Autodesk Inventor part; units mm, degrees
ref_plane "Work Plane1" through (6, 0, 0) normal (1, 0, 0) x (0, 0, -1)
ref_plane "YZ Plane" through (0, 0, 0) normal (1, 0, 0) x (0, 1, 0)
ref_plane "XZ Plane" through (0, 0, 0) normal (0, 1, 0) x (-1, 0, 0)
sketch "Sketch2" plane through (0, 0, 0) normal (1, 0, 0) x (0, 1, 0)
  line L0 (0, 0) -> (15, 0)
  line L1 (15, 0) -> (15, -10)
  line L2 (15, -10) -> (0, -10)
  line L3 (0, -10) -> (0, 0)
  dimension "d4" = 15
  dimension "d5" = 10
extrude "Extrusion2" add sketch "Sketch2" along normal blind 12
sketch "Sketch3" plane through (0, 0, 0) normal (0, 0, 1) x (1, 0, 0)
  line L0 (0, 0) -> (1, 0)
  line L1 (0, 0) -> (12, 0)
  line L2 (1, 0) -> (1, 13.5)
  line L3 (1, 13.5) -> (11, 13.5)
  line L4 (11, 13.5) -> (11, 0)
  line L5 (11, 0) -> (1, 0)
  dimension "d8" = 1
  dimension "d9" = 13.5
  dimension "d10" = 10
extrude "Extrusion3" cut sketch "Sketch3" against normal blind 8
sketch "Sketch4" plane through (0, 0, -10) normal (0, 0, -1) x (-1, 0, 0)
  line L0 (0, 15) -> (-12, 15)
  line L1 (0, 0) -> (-12, 0)
  line L2 (-12, 15) -> (0, 15)
  line L3 (0, 15) -> (0, 0)
  line L4 (0, 0) -> (-12, 0)
  line L5 (-12, 0) -> (-12, 15)
extrude "Extrusion4" add sketch "Sketch4" along normal blind 2
sketch "Sketch5" plane through (0, 0, -8) normal (0, 0, 1) x (1, 0, 0)
  line L0 (1, 13.5) -> (11, 13.5)
  line L1 (6, 13.5) -> (6, 10)
  line L2 (6, 10) -> (6, 3.5)
  circle A0 centre (6, 10) radius 1.2295
  circle A1 centre (6, 3.5) radius 1.2295
  point P0 (0, 0)
  dimension "d15" = 3.5
  dimension "d16" = 6.5
  dimension "d17" = 2.459
  dimension "d18" = 2.459
extrude "Extrusion5" cut sketch "Sketch5" against normal blind 4
sketch "Sketch6" plane through (0, 0, -8) normal (0, 0, 1) x (1, 0, 0)
  circle A0 centre (6, 10) radius 1.2295
  circle A1 centre (6, 10) radius 2.7
  circle A2 centre (6, 3.5) radius 1.2295
  circle A3 centre (6, 3.5) radius 2.7
  point P0 (0, 0)
  dimension "d21" = 5.4
  dimension "d22" = 5.4
extrude "Extrusion6" cut sketch "Sketch6" against normal blind 1.1
sketch "Sketch15" plane through (12, 0, 0) normal (1, 0, 0) x (0, 0, -1)
  line L0 (0, 15) -> (12, 15)
  line L1 (12, 15) -> (12, 0)
  line L2 (0, 15) -> (12, 15)
  line L3 (12, 15) -> (12, 0)
  line L4 (12, 0) -> (0, 0)
  line L5 (0, 0) -> (0, 15)
extrude "Extrusion14" add sketch "Sketch15" along normal blind 4
ref_plane "Work Plane1" through (6, 0, 0) normal (1, 0, 0) x (0, 0, -1)
mirror "Mirror1" about plane through (6, 0, 0) normal (1, 0, 0) of "Extrusion14"
sketch "Sketch16" plane through (1, 0, -8) normal (0, -1, 0) x (1, 0, 0)
  line L0 (10, 0) -> (0, 0)
  line L1 (5, 0) -> (7.5, 0)
  line L2 (7.5, 0) -> (7.5, -4)
  line L3 (-5, -4) -> (15, -4)
  line L4 (7.5, -4) -> (2.5, -4)
  line L5 (2.5, -4) -> (2.5, 0)
  line L6 (2.5, 0) -> (5, 0)
  point P0 (-1, 8)
  dimension "d61" = 2.5
  dimension "d62" = 4
  dimension "d63" = 5
  dimension "d64" = 4
extrude "Extrusion15" add sketch "Sketch16" along normal blind 10
sketch "Sketch18" plane through (0, 0, -12) normal (0, 0, -1) x (-1, 0, 0)
  line L0 (-16, 15) -> (4, 15)
  line L1 (4, 0) -> (-3.5, 0)
  line L2 (-16, 15) -> (4, 15)
  line L3 (4, 15) -> (4, 0)
  line L4 (4, 0) -> (-16, 0)
  line L5 (-16, 0) -> (-16, 15)
  line L6 (-8.5, -10) -> (-3.5, -10)
  line L7 (-3.5, 0) -> (-8.5, 0)
  line L8 (-8.5, 0) -> (-8.5, -10)
  line L9 (-8.5, -10) -> (-3.5, -10)
  line L10 (-3.5, -10) -> (-3.5, 0)
  circle A0 centre (-6, 3.5) radius 1.2295
  circle A1 centre (-6, 3.5) radius 1.2295
  circle A2 centre (-6, 10) radius 1.2295
  circle A3 centre (-6, 10) radius 1.2295
  point P0 (0, 0)
extrude "Extrusion16" add sketch "Sketch18" along normal blind 1
sketch "Sketch19" plane through (16, 0, 0) normal (1, 0, 0) x (0, 0, -1)
  line L0 (0, 15) -> (13, 15)
  line L1 (0, 15) -> (0, 40)
  line L2 (13, 45) -> (13, 15)
  line L3 (0, 57) -> (-10, 57)
  line L4 (0, 57) -> (13, 45)
  arc A0 (0, 40) -> (-5, 45) centre (-5, 40) ccw
  line L5 (-5, 45) -> (-10, 45)
  line L6 (-7, 51) -> (-10, 57)
  line L7 (-7, 51) -> (-10, 45)
  point P0 (0, 0)
  point P1 (0, 45)
  dimension "d69" = 30
  dimension "d75" = 5
  dimension "d76" = 5
extrude "Extrusion17" add sketch "Sketch19" against normal blind 20
properties part number "3point finger"
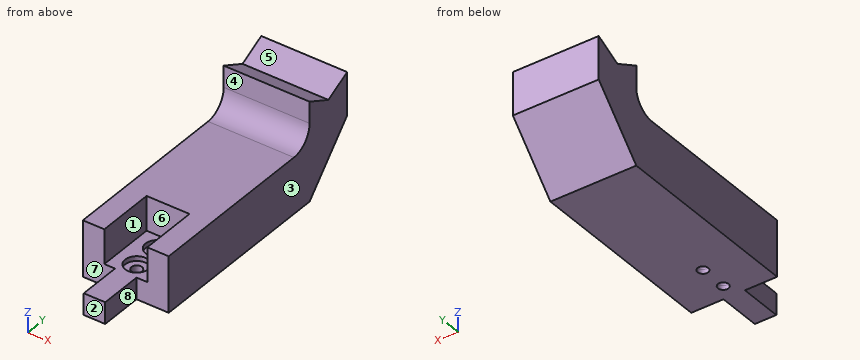
Design review of the part built by this model. Coordinates are the model's own, in mm. Face numbers are marked on the shaded views. A direction names the side the tool comes from. Give positions to 0.01 mm unless a question says otherwise; leave off trailing zeros. Loops run counter-clockwise (first coordinate to the right, second up) from the corner with the lowest first, then second, coordinate; pieces in that order, holes last. Notation, with made-up numbers: M 15,14.25 L 29,14.25 A36 ccw 29,53.25 Z; hole C 71.5,31 d9. An arc over 180 degrees is marked long. Return JSON: item names as keys, results as strings. Group by question number.
Item 1: We need section B-B (y = 3.5). Give the boundary of the cut face in (x, z).
Item 2: Mouldability with a two-part tool opening along X and no side actions: class the marked faces 1, 2 and 3 as released by +X, released by -X, zero draft, split by the parting line, or undercut.
Item 3: We need section C-C (x = -0.75). Give the boundary of the cut face in (y, z), and give its area (3 significant figures).
Item 4: For probe 1 along X at (y, z) = (3.5, -12.55); probe 2 along Y at (x, z) = (6, -12.25); probe 3 along Y at (x, z) = (6, -11.3), list the stretches that pass through material, from the lowest coordinate up.
Item 5: Tool access review of the marked faces 4, 5, 6, 7 and 8: name each direction out of +Z, -Z, +X, -X, +Y, -Y from which nothing blocks a thin tool from reaching the whole face with its end or side.
Item 6: We need section D-D (z = -5). Give the boundary of the cut face in (x, y).
Item 7: Insertion check: pin 1 Ø2 at (x, y) = (13.5, 43.5) entering from +Z; pin 2 Ø4.5 at (x, y) = (6, 10) entering from +Z; pin 3 Ø6 at (x, z) = (0.5, 4) entering from -Y. Each pin has a flat end and moves straight along its axis. Give the tip position at first contact, or say it passes through.
Item 8: We need section A-A (z = 8). Give the boundary of the cut face in (x, y), and give its area (3 significant figures).
Output:
{
 "1": {"outline": "M -4,-13 L 4.77,-13 L 4.77,-9.1 L 3.3,-9.1 L 3.3,-8 L 1,-8 L 1,0 L -4,0 Z; M 7.23,-13 L 16,-13 L 16,0 L 11,0 L 11,-8 L 8.7,-8 L 8.7,-9.1 L 7.23,-9.1 Z"},
 "2": {"face 1": "undercut", "face 2": "zero draft", "face 3": "released by +X"},
 "3": {"outline": "M 0,-13 L 45,-13 L 57,0 L 57,10 L 51,7 L 45,10 L 45,5 A5 cw 40,0 L 0,0 Z", "area": "770 mm^2"},
 "4": {"probe 1": "x = -4 to 4.77, 7.23 to 16", "probe 2": "y = -10 to 2.27, 4.73 to 8.77, 11.23 to 45.69", "probe 3": "y = -10 to 2.27, 4.73 to 8.77, 11.23 to 46.57"},
 "5": {"face 4": "+Z, +X, -X, -Y", "face 5": "+Z, +X, -X", "face 6": "+Z, -Y", "face 7": "+Z, -Z, -X, -Y", "face 8": "+Z, -Z, +X, -Y"},
 "6": {"outline": "M -4,0 L 1,0 L 1,13.5 L 11,13.5 L 11,0 L 16,0 L 16,52.38 L -4,52.38 Z"},
 "7": {"pin 1": "stops at z = 2.82", "pin 2": "stops at z = -9.1", "pin 3": "stops at y = 43"},
 "8": {"outline": "M -4,45 L 16,45 L 16,49 L -4,49 Z; M -4,53 L 16,53 L 16,57 L -4,57 Z", "area": "160 mm^2"}
}
